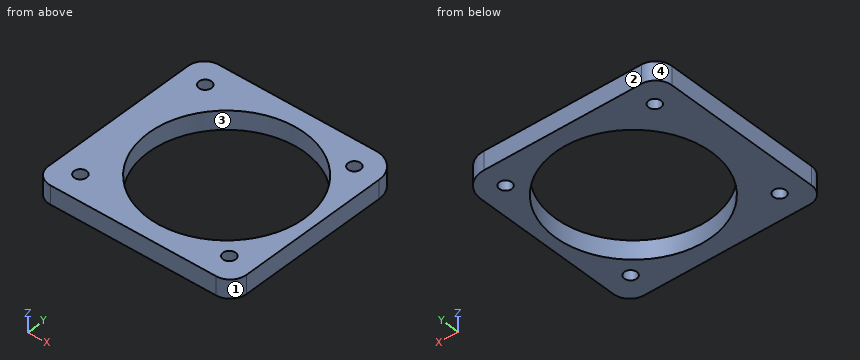
from build123d import *

# Parameters (mm, degrees)
F0_R     = 3.175
F0_R_2   = 39.878
F1_DEPTH = 9.525


with BuildPart() as f1:
    # F0 (on Top) → F1 (new body)
    with BuildSketch(Plane.XY):
        with BuildLine():
            Line((38.1, 49.2125), (-42.389483, 49.2125))
            ThreePointArc((-42.389483, 49.2125), (-48.246814, 46.786314), (-50.673, 40.928983))
            Line((-50.673, 40.928983), (-50.673, -40.928983))
            ThreePointArc((-50.673, -40.928983), (-48.246814, -46.786314), (-42.389483, -49.2125))
            Line((-42.389483, -49.2125), (42.389483, -49.2125))
            ThreePointArc((42.389483, -49.2125), (48.246814, -46.786314), (50.673, -40.928983))
            Line((50.673, -40.928983), (50.673, 36.6395))
            ThreePointArc((50.673, 36.6395), (46.990454, 45.529954), (38.1, 49.2125))
        make_face()
        with Locations((-38.1, -36.5125)):
            Circle(F0_R, mode=Mode.SUBTRACT)
        with Locations((38.1, -36.5125)):
            Circle(F0_R, mode=Mode.SUBTRACT)
        with Locations((-38.1, 36.5125)):
            Circle(F0_R, mode=Mode.SUBTRACT)
        with Locations((4.7752, 0)):
            Circle(F0_R_2, mode=Mode.SUBTRACT)
        with Locations((38.1, 36.6395)):
            Circle(F0_R, mode=Mode.SUBTRACT)
    extrude(amount=F1_DEPTH)


solid = f1.part
Read the model definition and answer for the solid it produces. Units are mm, in the model's axes. Face numbers are marked on the shaded views. Coordinates: 2 decimals unless noted, no trailing zeros. Loops run counter-clockwise (first coordinate to the right, second up) from the corner with the lowest first, then second, coordinate; pieces in that order, holes last.
Q1. The part is cut by section A-A on x = -38.1. Write down the section's boundary in (y, z) (1 decimal).
Q2. The mould has two halves that part along X. Classify the marked faces 1, 2, 3 and 4: +X half, -X half, draft (parallel to the pull), parting line (faces both ways), or undercut.
Q3. The part is cut by section D-D on x = 24. Write down the section's boundary in (y, z) (1 decimal), and give its area (3 significant figures).
Q4. This flat-tipped pin is pushed along its axis until it touches: pin 1 Ø4 at (x, y) = (38.1, -36.51) entering from +Z. Where does it stop, or does it pass through?
Q5. Consider probe 1 along Y at (x, z) = (-38.1, 2); probe 2 along Y at (x, z) = (38.1, 5.5); probe 3 along Y at (x, z) = (4.5, 8.25). Determine where each line is inside the solid, lowest interval first.
Q6. The part is cut by section C-C on z = 6.5. Give the number of separate pieces and of enclosed holes in the cut face, and give its area (3 significant figures).
Q7. The part is cut by section B-B on y = 0. Write down the section's boundary in (x, z) (3 decimals), and give its area (3 significant figures).
Results below:
1. outline: (-49.2, 0) - (-39.7, 0) - (-39.7, 9.5) - (-49.2, 9.5) - close; (-33.3, 0) - (33.3, 0) - (33.3, 9.5) - (-33.3, 9.5) - close; (39.7, 0) - (49.2, 0) - (49.2, 9.5) - (39.7, 9.5) - close
2. face 1: +X half
2. face 2: draft
2. face 3: undercut
2. face 4: -X half
3. outline: (-49.2, 0) - (-34.9, 0) - (-34.9, 9.5) - (-49.2, 9.5) - close; (34.9, 0) - (49.2, 0) - (49.2, 9.5) - (34.9, 9.5) - close
3. area: 272 mm2
4. pin 1: passes through
5. probe 1: y = -49.21 to -39.69, -33.34 to 33.34, 39.69 to 49.21
5. probe 2: y = -49.21 to -39.69, -33.34 to -21.9, 21.9 to 33.46, 39.81 to 49.21
5. probe 3: y = -49.21 to -39.88, 39.88 to 49.21
6. separate pieces: 1
6. enclosed holes: 5
6. area: 4,770 mm2
7. outline: (-50.673, 0) - (-35.103, 0) - (-35.103, 9.525) - (-50.673, 9.525) - close; (44.653, 0) - (50.673, 0) - (50.673, 9.525) - (44.653, 9.525) - close
7. area: 206 mm2
